Input: part model. Units: mm. Frame: model coordinates. A direction names the side the tool comes from. Round coordinates to 2 decimals unless told otherwise and drop trailing zeros. Loops run counter-clockwise (first coordinate to the right, second up) from the corner with the lowest first, then second, coordinate; pieces in that order, holes last. Notation, with made-up numbers: (-36.75, -6.75) - (22.25, -6.75) arc R32 cw to (22.25, 31.25) - close; hole circle Ø2 at (-31, 13). An arc over 180 degrees is marked (long way). One line per question, with ' | ' between items. Start each with the question number.
Item 1: Section A-A, the plane x = 0. Return loops of the section in (y, z) (3 decimals).
Item 2: Set-up query: faces 1 (the face through (-7.559, 10.279, -5.796)), 2 (the face through (0, 11.887, 0)), 3 (the face through (4, 7.925, 0)). Return all of +Z, -Z, +X, -X, +Y, -Y with unobstructed straight access to the full face (end or side cutting, diameter ignored); none if empty.
Item 3: Draft query along X for faces 4 (the face through (-0.69, 4.39, 3.1)), 5 (the face through (0.787, 13, 0)), 6 (the face through (0, 0, 0)). Return one class per face: pulls with the +X half, pulls with the -X half, needs draft (parallel to the pull), parting line crosses it, or undercut.
Item 4: First-contact query: pin 1 (2 mm diameter, centred on y = 2.5, z = -2.5, fed in from +X); pin 2 (4 mm diameter, centred on y = 2, z = 7, fed in from -X); pin 3 (8 mm diameter, centred on x = -3, z = -2, fed in from -Y); pin 4 (5 mm diameter, centred on x = -6.5, y = 6, fed in from -Z). Flat tips, straight axial feed; report the tip coordinate or a pass-through.
Item 5: Section C-C, the plane y = 2. Return loops of the section in (x, z) (3 decimals), plus the area to 3 significant figures.
Item 6: Section B-B, the plane z = 0. Return loops of the section in (x, y) (3 decimals).
Item 7: Material intervals for line 1 along Y through (x, z) = (-0.5, -4.25); line 2 along X through (y, z) = (12.25, -8); line 3 along Y through (x, z) = (0, 1.25), sorted ascending.
Autodesk Inventor part; units mm, degrees
ref_plane "Work Plane1" through (0, 14.2748, 0) normal (0, -1, 0) x (1, 0, 0)
ref_plane "YZ Plane" through (0, 0, 0) normal (1, 0, 0) x (0, 1, 0)
ref_plane "XZ Plane" through (0, 0, 0) normal (0, 1, 0) x (-1, 0, 0)
sketch "Sketch1" plane through (0, 0, 0) normal (0, 0, 1) x (1, 0, 0)
  line L0 (0, 0) -> (19.05, 0)
  line L1 (-9.525, 7.9248) -> (9.525, 7.9248)
  line L2 (-9.525, 7.9248) -> (-9.525, 12.7)
  line L3 (-9.525, 12.7) -> (9.525, 12.7)
  line L4 (9.525, 12.7) -> (9.525, 7.9248)
  line L5 (0, 12.7) -> (0, 14.2748)
  arc A0 (9.525, 12.7) -> (-9.525, 12.7) centre (0, -15.318) ccw
  line L6 (0, 7.9248) -> (0, 0)
  line L7 (3.175, 0) -> (3.175, 7.9248)
  line L8 (3.175, 0) -> (-3.175, 0)
  line L9 (-3.175, 0) -> (-3.175, 7.9248)
  line L10 (-15.24, 0) -> (24.765, 0)
  line L11 (0, -21.2366) -> (0, 20.1934)
  dimension "d1" = 19.05
  dimension "d2" = 4.7752
  dimension "d4" = 1.5748
  dimension "d6" = 3.175
  dimension "d7" = 6.35
  dimension "d19" = 14.2748
revolve "Revolution1" add sketch "Sketch1" angle 360 about axis through (0, -10, 0) along (0, 1, 0) picked at (5.3129, 12.9905) contours L6 L1 L7 L0 | L11 L3 L4 L1 | L5 A0 L3
ref_plane "Work Plane1" through (0, 14.2748, 0) normal (0, -1, 0) x (1, 0, 0)
sketch "Sketch2" plane through (0, 14.2748, 0) normal (0, -1, 0) x (1, 0, 0)
  circle A0 centre (0, 0) radius 9.525
  line L0 (0.7874, 9.4924) -> (0.7874, -9.4924)
  line L1 (-0.7874, 9.4924) -> (-0.7874, -9.4924)
  line L2 (0, -13.335) -> (0, 13.335)
  line L3 (-13.335, 0) -> (13.335, 0)
  point P0 (0, 9.525)
  dimension "d11" = 1.5748
extrude "Extrusion1" cut sketch "Sketch2" along normal blind 2.3876 contours L0 L3 L2 A0 | A0 L2 L3 L0 | L2 L3 L1 A0 | A0 L1 L3 L2
chamfer "Chamfer1" distance 0.762 angle 45 1 edges at (-3.175, 0, 0)
thread "Thread1"
properties part number "Ch7(5) Part 12 Screw NEED TO DO"
Return value:
1) outline: (0, -2.413) - (0.762, -3.175) - (7.925, -3.175) - (7.925, -9.525) - (11.887, -9.525) - (11.887, 9.525) - (7.925, 9.525) - (7.925, 3.175) - (0.762, 3.175) - (0, 2.413) - close
2) face 1: +Y, -Y | face 2: +Z, -Z, +Y | face 3: -Y
3) face 4: parting line crosses it | face 5: undercut | face 6: needs draft
4) pin 1: x = 2.8 | pin 2: through | pin 3: y = 0 | pin 4: z = -8.17
5) outline: circle Ø6.35 at (0, 0) | area: 31.7 mm2
6) outline: (-9.525, 7.925) - (-3.175, 7.925) - (-3.175, 0.762) - (-2.413, 0) - (2.413, 0) - (3.175, 0.762) - (3.175, 7.925) - (9.525, 7.925) - (9.525, 12.7) arc R29.593 ccw to (0.787, 14.264) - (0.787, 11.887) - (-0.787, 11.887) - (-0.787, 14.264) arc R29.593 ccw to (-9.525, 12.7) - close
7) line 1: 7.92 to 11.89 | line 2: -5.17 to -0.79, 0.79 to 5.17 | line 3: 0 to 11.89
